Check sheet for the modelled part. Datum: model origin and axes. Units: mm. A direction names the side the tool comes from. Give positions to 0.01 mm unless a question says otherwise; leave off trailing zeros. Write each loop counter-clockwise with the first axis right and the second up, starting at its lowest first coordinate (ties: lowest second). Pieces come first, ordered by that corner, then holes. Notation, with made-up numbers: (-7.5, 11) -> (41.5, 11) arc R24 cw to (41.5, 23) -> close; hole circle Ø11 at (35.5, 45). An arc over 180 degrees is marked (long way). Answer as a JSON object with one key per item and string values.
from build123d import *

# Parameters (mm, degrees)
SKETCH1_W           = 549.631
SKETCH1_H           = 749.631
BOSS_EXTRUDE1_DEPTH = 933.333333333
SKETCH2_W           = 449.8
SKETCH2_H           = 649.8
BOSS_EXTRUDE2_DEPTH = 933.333333333
SKETCH3_W           = 349.969
SKETCH3_H           = 549.969
BOSS_EXTRUDE3_DEPTH = 933.333333333


with BuildPart() as part:
    # Sketch1 → Boss-Extrude1 (new body)
    with BuildSketch(Plane(origin=(0, 0, 0), x_dir=(0, 0, -1), z_dir=(1, 0, 0))):
        Rectangle(SKETCH1_W, SKETCH1_H)
    extrude(amount=BOSS_EXTRUDE1_DEPTH)

    # Sketch2 → Boss-Extrude2 (add)
    with BuildSketch(Plane(origin=(933.333333333, 0, 0), x_dir=(0, 0, -1), z_dir=(1, 0, 0))):
        Rectangle(SKETCH2_W, SKETCH2_H)
    extrude(amount=BOSS_EXTRUDE2_DEPTH)

    # Sketch3 → Boss-Extrude3 (add)
    with BuildSketch(Plane(origin=(1866.666666667, 0, 0), x_dir=(0, 0, -1), z_dir=(1, 0, 0))):
        Rectangle(SKETCH3_W, SKETCH3_H)
    extrude(amount=BOSS_EXTRUDE3_DEPTH)


solid = part.part
1. Access from +Z, -Z, +X, -X, +Y, -Y to the whole of each face (thin tool, end or side, straight path). Record for faces 1 (the face through (1393, -5, -224.9)), 2 (the face through (2327, 274.984, 2)), 3 (the face through (1393, -324.9, 3)), 4 (the face through (1393, -5, 224.9)).
Determined:
{"face 1": "-Z, +X, +Y, -Y", "face 2": "+Z, -Z, +X, +Y", "face 3": "+Z, -Z, +X, -Y", "face 4": "+Z, +X, +Y, -Y"}
2. Sectioned sample at A-A, the plane y = -187.5. Enter the section's corners in (x, z).
Determined:
{"outline": "(0, -274.82) -> (933.33, -274.82) -> (933.33, -224.9) -> (1866.67, -224.9) -> (1866.67, -174.98) -> (2800, -174.98) -> (2800, 174.98) -> (1866.67, 174.98) -> (1866.67, 224.9) -> (933.33, 224.9) -> (933.33, 274.82) -> (0, 274.82) -> close"}
3. Sectioned sample at C-C, the plane x = 1962. Enter the section's corners in (y, z).
Determined:
{"outline": "(-274.98, -174.98) -> (274.98, -174.98) -> (274.98, 174.98) -> (-274.98, 174.98) -> close"}
4. Scan lines: L1, parallel to Y at x = 2287.5, z = 122; L2, parallel to Z at x = 2450, y = 180; L3, parallel to X at y = 271.5, z = -190. Record each from-to range of solid material in increasing order. Write a range as [from, to].
Determined:
{"L1": "[-274.98, 274.98]", "L2": "[-174.98, 174.98]", "L3": "[0, 1866.67]"}
5. Go/stop test with flat-tipped pins: P1, Ø5, axis at x = 1112.5, y = 147, coming from the -Z side; P2, Ø2, axis at x = 1855.5, z = 10, coming from the +Y side; P3, Ø3, axis at x = 1655.5, y = -218.5, coming from the +Z side; P4, Ø5, axis at y = -2.5, z = 4, coming from the -X side. Record where each tip stops, or that it passes through.
Determined:
{"P1": "z = -224.9", "P2": "y = 324.9", "P3": "z = 224.9", "P4": "x = 0"}
6. Sectioned sample at D-D, the plane x = 1583.5. Enter the section's corners in (y, z), plus the area to 3 significant figures.
Determined:
{"outline": "(-324.9, -224.9) -> (324.9, -224.9) -> (324.9, 224.9) -> (-324.9, 224.9) -> close", "area": "292,000 mm^2"}
7. Sectioned sample at B-B, the plane z = -137.5. Enter the section's corners in (x, y).
Determined:
{"outline": "(0, -374.82) -> (933.33, -374.82) -> (933.33, -324.9) -> (1866.67, -324.9) -> (1866.67, -274.98) -> (2800, -274.98) -> (2800, 274.98) -> (1866.67, 274.98) -> (1866.67, 324.9) -> (933.33, 324.9) -> (933.33, 374.82) -> (0, 374.82) -> close"}
